CAD build for the part. Positions are in the model's coordinates, mm. Give positions to 0.01 mm unless a question says otherwise; leave off trailing zeros. Order: outer loops, then holes, each group sorted by start corner. A loop starts at its lowest first (then second) coordinate and runs counter-clockwise, first axis right, second up.
```python
from build123d import *

# Parameters (mm, degrees)
BOSS_EXTRUDE1_DEPTH = 2.54
CUT_EXTRUDE1_START  = -3.54
SKETCH2_R           = 0.635
CUT_EXTRUDE1_DEPTH  = 4.54


with BuildPart() as part:
    # Sketch1 → Boss-Extrude1 (new body)
    with BuildSketch(Plane.XY):
        with BuildLine():
            Line((0, 2.54), (25.4, 2.54))
            ThreePointArc((25.4, 2.54), (27.94, 0), (25.4, -2.54))
            Line((25.4, -2.54), (0, -2.54))
            ThreePointArc((0, -2.54), (-2.54, 0), (0, 2.54))
        make_face()
    extrude(amount=BOSS_EXTRUDE1_DEPTH)

    # Sketch2 → Cut-Extrude1 (cut)
    with BuildSketch(Plane.XY.offset(2.54).offset(CUT_EXTRUDE1_START)):
        Circle(SKETCH2_R)
    cut_extrude1 = extrude(amount=CUT_EXTRUDE1_DEPTH, mode=Mode.SUBTRACT)

    # Mirror1: Cut-Extrude1 across plane
    add(cut_extrude1.mirror(Plane(origin=(12.7, 0, 0), x_dir=(0, 0, 1), z_dir=(1, 0, 0))), mode=Mode.SUBTRACT)


solid = part.part
```
Item 1: Wall check: L1, parallel to Y at x = 25.4, z = 1.8 (3 decimals); L2, parallel to X at y = -0.45, z = 0.65; L3, parallel to Y at x = -0.5, z = 1.7. Give the ranges that are in metal, low to high.
Item 2: Slice it at B-B (z = 0.7). Give the cut face in (x, y) (3 decimals).
Item 3: Slice it at D-D (y = 1.75). Give the cut face in (x, z).
Item 4: Slice it at A-A (y = 0). Give the cut face in (x, z) (3 decimals).
Item 5: Two-plate mould, pull along Y, no slides. Class faces 1 (the face through (13, 2.54, 1)), 2 (the face through (24.81, -0.24, 1.25)), 3 (the face through (27.94, 0.06, 1.25)): released by +Y, released by -Y, zero draft, split by the parting line, or undercut.
Item 6: Slice it at C-C (y = -1.15). Give the cut face in (x, z).
A:
1. L1: y = -2.54 to -0.635, 0.635 to 2.54
1. L2: x = -2.5 to -0.45, 0.45 to 24.95, 25.85 to 27.9
1. L3: y = -2.49 to -0.39, 0.39 to 2.49
2. outline: (0, -2.54) - (25.4, -2.54) arc R2.54 ccw to (25.4, 2.54) - (0, 2.54) arc R2.54 ccw to start; hole circle Ø1.27 at (0, 0); hole circle Ø1.27 at (25.4, 0)
3. outline: (-1.84, 0) - (27.24, 0) - (27.24, 2.54) - (-1.84, 2.54) - close
4. outline: (-2.54, 0) - (-0.635, 0) - (-0.635, 2.54) - (-2.54, 2.54) - close; (0.635, 0) - (24.765, 0) - (24.765, 2.54) - (0.635, 2.54) - close; (26.035, 0) - (27.94, 0) - (27.94, 2.54) - (26.035, 2.54) - close
5. face 1: released by +Y
5. face 2: undercut
5. face 3: split by the parting line
6. outline: (-2.26, 0) - (27.66, 0) - (27.66, 2.54) - (-2.26, 2.54) - close
